Design review of the part built by this model. Coordinates are the model's own, in mm. Coordinates: 2 decimals unless noted, no trailing zeros. Return JSON: item names as keys, results as strings. Group by question number.
Autodesk Inventor part; units mm, degrees
ref_plane "to_frame_XY" through (0, 0, 0) normal (0, 0, 1) x (1, 0, 0)
ref_plane "to_frame_YZ" through (0, 0, 0) normal (1, 0, 0) x (0, 1, 0)
ref_plane "to_frame_ZX" through (0, 0, 0) normal (0, 1, 0) x (0, 0, 1)
sketch "Sketch_5" plane through (0, 0, 0) normal (0, 0, 1) x (1, 0, 0)
  arc A0 (-10, 3.3) -> (-9.7, 3) centre (-9.7, 3.3) ccw
  line L0 (-9.7, 3) -> (-8, 3)
  line L1 (-8, 3) -> (-8, 6)
  line L2 (-8, 6) -> (-7.0607, 6)
  line L3 (-7.0607, 6) -> (-4, 2.9393)
  line L4 (-4, 2.9393) -> (-4, 0.3)
  line L5 (-4, 0.3) -> (-3.7, 0)
  line L6 (-3.7, 0) -> (-4, -0.3)
  line L7 (-4, -0.3) -> (-4, -2.9393)
  line L8 (-4, -2.9393) -> (-7.0607, -6)
  line L9 (-7.0607, -6) -> (-8, -6)
  line L10 (-8, -6) -> (-8, -3)
  line L11 (-8, -3) -> (-9.7, -3)
  arc A1 (-9.7, -3) -> (-10, -3.3) centre (-9.7, -3.3) ccw
  line L12 (-10, -3.3) -> (-10, -9)
  arc A2 (-10, -9) -> (-9, -10) centre (-9, -9) ccw
  line L13 (-9, -10) -> (-3.3, -10)
  arc A3 (-3.3, -10) -> (-3, -9.7) centre (-3.3, -9.7) ccw
  line L14 (-3, -9.7) -> (-3, -8)
  line L15 (-3, -8) -> (-6, -8)
  line L16 (-6, -8) -> (-6, -7.0607)
  line L17 (-6, -7.0607) -> (-2.9393, -4)
  line L18 (-2.9393, -4) -> (-0.3, -4)
  line L19 (-0.3, -4) -> (0, -3.7)
  line L20 (0, -3.7) -> (0.3, -4)
  line L21 (0.3, -4) -> (2.9393, -4)
  line L22 (2.9393, -4) -> (6, -7.0607)
  line L23 (6, -7.0607) -> (6, -8)
  line L24 (6, -8) -> (3, -8)
  line L25 (3, -8) -> (3, -9.7)
  arc A4 (3, -9.7) -> (3.3, -10) centre (3.3, -9.7) ccw
  line L26 (3.3, -10) -> (9, -10)
  arc A5 (9, -10) -> (10, -9) centre (9, -9) ccw
  line L27 (10, -9) -> (10, -3.3)
  arc A6 (10, -3.3) -> (9.7, -3) centre (9.7, -3.3) ccw
  line L28 (9.7, -3) -> (8, -3)
  line L29 (8, -3) -> (8, -6)
  line L30 (8, -6) -> (7.0607, -6)
  line L31 (7.0607, -6) -> (4, -2.9393)
  line L32 (4, -2.9393) -> (4, -0.3)
  line L33 (4, -0.3) -> (3.7, 0)
  line L34 (3.7, 0) -> (4, 0.3)
  line L35 (4, 0.3) -> (4, 2.9393)
  line L36 (4, 2.9393) -> (7.0607, 6)
  line L37 (7.0607, 6) -> (8, 6)
  line L38 (8, 6) -> (8, 3)
  line L39 (8, 3) -> (9.7, 3)
  arc A7 (9.7, 3) -> (10, 3.3) centre (9.7, 3.3) ccw
  line L40 (10, 3.3) -> (10, 9)
  arc A8 (10, 9) -> (9, 10) centre (9, 9) ccw
  line L41 (9, 10) -> (3.3, 10)
  arc A9 (3.3, 10) -> (3, 9.7) centre (3.3, 9.7) ccw
  line L42 (3, 9.7) -> (3, 8)
  line L43 (3, 8) -> (6, 8)
  line L44 (6, 8) -> (6, 7.0607)
  line L45 (6, 7.0607) -> (2.9393, 4)
  line L46 (2.9393, 4) -> (0.3, 4)
  line L47 (0.3, 4) -> (0, 3.7)
  line L48 (0, 3.7) -> (-0.3, 4)
  line L49 (-0.3, 4) -> (-2.9393, 4)
  line L50 (-2.9393, 4) -> (-6, 7.0607)
  line L51 (-6, 7.0607) -> (-6, 8)
  line L52 (-6, 8) -> (-3, 8)
  line L53 (-3, 8) -> (-3, 9.7)
  arc A10 (-3, 9.7) -> (-3.3, 10) centre (-3.3, 9.7) ccw
  line L54 (-3.3, 10) -> (-9, 10)
  arc A11 (-9, 10) -> (-10, 9) centre (-9, 9) ccw
  line L55 (-10, 9) -> (-10, 3.3)
  circle A12 centre (0, 0) radius 2.1
extrude "Extrusion1" add sketch "Sketch_5" against normal blind 1000
ref_plane "to_frame_XY" through (0, 0, 0) normal (0, 0, 1) x (1, 0, 0)
ref_plane "to_frame_YZ" through (0, 0, 0) normal (1, 0, 0) x (0, 1, 0)
ref_plane "to_frame_ZX" through (0, 0, 0) normal (0, 1, 0) x (0, 0, 1)
sketch "Sketch2" plane through (-10, -3.3, -1000) normal (-1, 0, 0) x (0, 0, 1)
  line L0 (-212.6604, -150.7885) -> (785, -150.7885)
  line L1 (785, -150.7885) -> (785, 147.9074)
  line L2 (785, 147.9074) -> (-212.6604, 147.9074)
  line L3 (-212.6604, 147.9074) -> (-212.6604, -150.7885)
  point P0 (1000, 3.3)
  dimension "d3" = 215
extrude "Extrusion2" cut sketch "Sketch2" against normal through all
equation "\"d0\" = L"
equation "\"L\" = 1000"
properties part number "KHFS5-2020-1000"
Item 1: The part is to be moulded in two halves that separate along Y. For faces 1 (the cylindrical face through (2.003, 0.631, -105.995)), 2 (the flat face through (6, 10, -106)), 3 (the flat face through (-0.1, 2.4, 0)), say which applies: pulls with the +Y half, pulls with the -Y half, needs draft (parallel to the pull), parting line crosses it, or undercut.
Item 2: For pin 1 (3 mm diameter, centred on x = 1, z = -102, fed in from -Y); pin 2 (5 mm diameter, centred on y = 0, z = -52.5, fed in from +X); pin 3 (1.3 mm diameter, centred on y = -2, z = -105, fed in from -X), all flat-tipped, find the tip position at first contact; note any pin that passes through.
Item 3: For line 1 (Y direction, x = -4.5, z = -9); line 2 (Y direction, x = -4.25, z = -93.5); line 3 (Y direction, x = 0, z = -148.5), list the stretches that pass through material, from the lowest coordinate up.
Geometry check:
{
 "1": {"face 1": "undercut", "face 2": "pulls with the +Y half", "face 3": "needs draft"},
 "2": {"pin 1": "y = -4", "pin 2": "x = 4", "pin 3": "x = -4"},
 "3": {"line 1": "-10 to -8, -5.56 to -3.44, 3.44 to 5.56, 8 to 10", "line 2": "-10 to -8, -5.31 to -3.19, 3.19 to 5.31, 8 to 10", "line 3": "-3.7 to -2.1, 2.1 to 3.7"}
}
